For this review, take the finished solid that the model builds, in its own axes (mm). Face numbers are marked on the shaded views. A direction names the side the tool comes from. Coordinates: 2 decimals unless noted, no trailing zeros. Loops run counter-clockwise (first coordinate to the right, second up) from the corner with the lowest first, then second, coordinate; pieces in that order, holes last. Notation, with made-up numbers: (34, -9.5) -> (40, -9.5) arc R38 ccw to (40, 28.5) -> close; hole circle Ø10 at (2.25, -7.75). An arc over 180 degrees is marked (long way). Use a Markdown table: item, result.
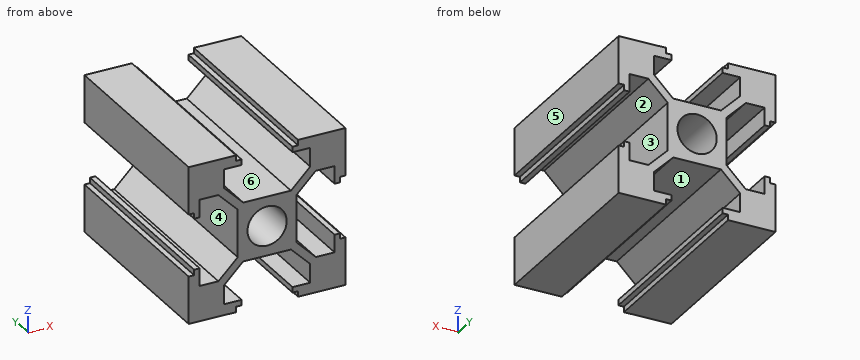
from build123d import *

# Parameters (mm, degrees)
F0_R     = 2.5
F1_DEPTH = 25


with BuildPart() as f1:
    # F0 (on Front) → F1 (new body)
    with BuildSketch(Plane.XZ):
        Polygon((10, 3.95), (10, 10), (3.95, 10), (3.95, 9.3), (3.25, 9.3), (3.25, 8.6), (5.5, 8.6), (5.5, 6.207107), (3.042893, 3.75), (0, 3.75), (-3.042893, 3.75), (-5.5, 6.207107), (-5.5, 8.6), (-3.25, 8.6), (-3.25, 9.3), (-3.95, 9.3), (-3.95, 10), (-10, 10), (-10, 3.95), (-9.3, 3.95), (-9.3, 3.25), (-8.6, 3.25), (-8.6, 5.5), (-6.207107, 5.5), (-3.75, 3.042893), (-3.75, 0), (-3.75, -3.042893), (-6.207107, -5.5), (-8.6, -5.5), (-8.6, -3.25), (-9.3, -3.25), (-9.3, -3.95), (-10, -3.95), (-10, -10), (-3.95, -10), (-3.95, -9.3), (-3.25, -9.3), (-3.25, -8.6), (-5.5, -8.6), (-5.5, -6.207107), (-3.042893, -3.75), (0, -3.75), (3.042893, -3.75), (5.5, -6.207107), (5.5, -8.6), (3.25, -8.6), (3.25, -9.3), (3.95, -9.3), (3.95, -10), (10, -10), (10, -3.95), (9.3, -3.95), (9.3, -3.25), (8.6, -3.25), (8.6, -5.5), (6.207107, -5.5), (3.75, -3.042893), (3.75, 0), (3.75, 3.042893), (6.207107, 5.5), (8.6, 5.5), (8.6, 3.25), (9.3, 3.25), (9.3, 3.95), align=None)
        Circle(F0_R, mode=Mode.SUBTRACT)
    extrude(amount=F1_DEPTH)


solid = f1.part
(1) Take a section at C-C on x = 5. Write out the cut boundary in (y, z), plus the area to 3 significant figures.
Found:
| item | result |
|---|---|
| outline | (-25, -10) -> (0, -10) -> (0, -8.6) -> (-25, -8.6) -> close; (-25, -5.71) -> (0, -5.71) -> (0, -4.29) -> (-25, -4.29) -> close; (-25, 4.29) -> (0, 4.29) -> (0, 5.71) -> (-25, 5.71) -> close; (-25, 8.6) -> (0, 8.6) -> (0, 10) -> (-25, 10) -> close |
| area | 141 mm^2 |
(2) Take a section at A-A on x = 0. Write out the cut boundary in (y, z).
Found:
| item | result |
|---|---|
| outline | (-25, -3.75) -> (0, -3.75) -> (0, -2.5) -> (-25, -2.5) -> close; (-25, 2.5) -> (0, 2.5) -> (0, 3.75) -> (-25, 3.75) -> close |
(3) Take a section at B-B on z = 0. Write out the cut boundary in (x, y).
Found:
| item | result |
|---|---|
| outline | (-3.75, -25) -> (-2.5, -25) -> (-2.5, 0) -> (-3.75, 0) -> close; (2.5, -25) -> (3.75, -25) -> (3.75, 0) -> (2.5, 0) -> close |
(4) For pin 1 Ø1.5 at (y, z) = (-15, -1) entering from -X; pin 2 Ø4 at (y, z) = (-21.5, -0.5) entering from +X; pin 3 Ø0.8 at (x, y) = (-3.5, -16.5) entering from -Z, all flat-tipped, find the tip position at first contact; note any pin that passes through.
Found:
| item | result |
|---|---|
| pin 1 | stops at x = -3.75 |
| pin 2 | stops at x = 3.75 |
| pin 3 | stops at z = -9.3 |
(5) Mouldability with a two-part tool opening along Z and no side actions: class the marked faces 4, 5 and 6 as pulls with the +Z half, pulls with the -Z half, needs draft (parallel to the pull), parting line crosses it, or undercut.
Found:
| item | result |
|---|---|
| face 4 | undercut |
| face 5 | needs draft |
| face 6 | pulls with the +Z half |
(6) For the marked faces 1, 2 and 3, list the 3-axis set-ups (+Z, -Z, +X, -X, +Y, -Y) from which the entire face can be reached by the end or side of a thin tool; tool diameter is ignored.
Found:
| item | result |
|---|---|
| face 1 | -Z, +Y, -Y |
| face 2 | +Y, -Y |
| face 3 | +X, +Y, -Y |
(7) For line 1 along Z through (x, y) = (0, -9); line 2 along Z through (x, y) = (-4.75, -2.75); line 3 along X through (y, z) = (-2.5, 8.25), list the stretches that pass through material, from the lowest coordinate up.
Found:
| item | result |
|---|---|
| line 1 | z = -3.75 to -2.5, 2.5 to 3.75 |
| line 2 | z = -10 to -8.6, -5.46 to -4.04, 4.04 to 5.46, 8.6 to 10 |
| line 3 | x = -10 to -5.5, 5.5 to 10 |
